from build123d import *

# Parameters (mm, degrees)
BOSS_EXTRUDE1_DEPTH = 3
SKETCH3_W           = 23.052059357
SKETCH3_H           = 2.618596089
BOSS_EXTRUDE2_DEPTH = 20
SKETCH5_W           = 23.052059357
SKETCH5_H           = 27.381403911
BOSS_EXTRUDE3_DEPTH = 3


with BuildPart() as part:
    # Sketch2 → Boss-Extrude1 (new body)
    with BuildSketch(Plane(origin=(0, 0, -200), x_dir=(-1, 0, 0), z_dir=(0, 0, -1))):
        Polygon((91.240837696, 22.154450262), (91.240837696, -7.845549738), (68.188778339, -7.845549738), (68.188778339, 22.154450262), (68.188778339, 25.05163022), (91.240837696, 25.05163022), align=None)
    extrude(amount=BOSS_EXTRUDE1_DEPTH)

    # Sketch3 → Boss-Extrude2 (add)
    with BuildSketch(Plane.XY.offset(-200)):
        with Locations((-79.714808018, 20.845152218)):
            Rectangle(SKETCH3_W, SKETCH3_H)
    extrude(amount=BOSS_EXTRUDE2_DEPTH)

    # Sketch5 → Boss-Extrude3 (add)
    with BuildSketch(Plane.XY.offset(-180)):
        with Locations((-79.714808018, 5.845152217)):
            Rectangle(SKETCH5_W, SKETCH5_H)
    extrude(amount=-BOSS_EXTRUDE3_DEPTH)


solid = part.part
Here's how the part is built. I have some questions about the finished solid (model axes, mm). A direction names the side the tool comes from. Coordinates: 2 decimals unless noted, no trailing zeros. Write each loop counter-clockwise with the first axis right and the second up, starting at its lowest first coordinate (ties: lowest second). Pieces come first, ordered by that corner, then holes.
Item 1: Will these pins go through, and if not, where does the flat tip stop? pin 1 (4 mm diameter, centred on x = -88.5, z = -193.5, fed in from -Y); pin 2 (2 mm diameter, centred on y = 17, z = -192.5, fed in from +X); pin 3 (3 mm diameter, centred on x = -80.5, y = 24, fed in from +Z); pin 4 (1 mm diameter, centred on x = -78, z = -184, fed in from +Y).
Item 2: I want a section at D-D on z = -192.5. Write out the boundary of the cut face in (x, y).
Item 3: If I drill on line 1 (Z direction, x = -74.5, y = 18); line 2 (Y direction, x = -70, z = -192); line 3 (Y direction, x = -88.25, z = -181.25), over which ranges is the centre line in solid material (lowest first)?
Item 4: I want a section at C-C on z = -182.25. Write out the boundary of the cut face in (x, y).
Item 5: I want a section at B-B on x = -73.25. Write out the boundary of the cut face in (y, z), and give its area (3 significant figures).
Item 6: If we mould it in two halves opening along Z, with no side actions, what happens to faces 1 (the flat face through (-80, 19.536, -192)), 2 (the flat face through (-80, 25.052, -201)), 3 (the flat face through (-80, 24, -200))? For each: +Z half, -Z half, draft (parallel to the pull), parting line (faces both ways), or undercut.
Item 7: On a 3-axis mill with a long thin cutter (end or side, diameter ignored), from which of +Z, -Z, +X, -X, +Y, -Y can I reach the whole of each face in a straight line? I mean faces 4 (the flat face through (-91.241, 12, -182)), 5 (the flat face through (-80, 22.154, -190)), 6 (the flat face through (-80, 6, -200)). Say none if no direction works.
Item 8: I want a section at A-A on y = 6.5. Write out the boundary of the cut face in (x, z), and give its area (3 significant figures).
Findings below:
1. pin 1: stops at y = 19.54
1. pin 2: passes through
1. pin 3: stops at z = -200
1. pin 4: stops at y = 22.15
2. outline: (-91.24, 19.54) - (-68.19, 19.54) - (-68.19, 22.15) - (-91.24, 22.15) - close
3. line 1: z = -203 to -200, -183 to -180
3. line 2: y = 19.54 to 22.15
3. line 3: y = -7.85 to 22.15
4. outline: (-91.24, -7.85) - (-68.19, -7.85) - (-68.19, 22.15) - (-91.24, 22.15) - close
5. outline: (-7.85, -203) - (25.05, -203) - (25.05, -200) - (22.15, -200) - (22.15, -180) - (-7.85, -180) - (-7.85, -183) - (19.54, -183) - (19.54, -200) - (-7.85, -200) - close
5. area: 233 mm2
6. face 1: undercut
6. face 2: draft
6. face 3: +Z half
7. face 4: +Z, -Z, -X, +Y, -Y
7. face 5: +Z, +X, -X, +Y
7. face 6: +X, -X, -Y
8. outline: (-91.24, -203) - (-68.19, -203) - (-68.19, -200) - (-91.24, -200) - close; (-91.24, -183) - (-68.19, -183) - (-68.19, -180) - (-91.24, -180) - close
8. area: 138 mm2
